from build123d import *

# Parameters (mm, degrees)
SZKIC1_W                    = 22
SZKIC1_H                    = 37
DODANIE_WYCI_GNI_CIE1_DEPTH = 120
SZKIC2_W                    = 42
SZKIC2_H                    = 15
SZKIC2_W_2                  = 15
SZKIC2_H_2                  = 47
WYTNIJ_WYCI_GNI_CIE1_DEPTH  = 112
ZAOKR_GLENIE1_R             = 15
ZAOKR_GLENIE2_R             = 2


with BuildPart() as part:
    # Szkic1 → Dodanie-wyciągnięcie1 (new body)
    with BuildSketch(Plane.XY):
        Polygon((0, 0), (0, 100), (15, 100), (15, 53), (38, 53), (38, 15), (80, 15), (80, 0), align=None)
        with Locations((19, 26.5)):
            Rectangle(SZKIC1_W, SZKIC1_H, mode=Mode.SUBTRACT)
    extrude(amount=DODANIE_WYCI_GNI_CIE1_DEPTH)

    # Szkic2 → Wytnij-wyciągnięcie1 (cut)
    with BuildSketch(Plane.XY.offset(120)):
        with Locations((59, 7.5)):
            Rectangle(SZKIC2_W, SZKIC2_H)
        with Locations((7.5, 76.5)):
            Rectangle(SZKIC2_W_2, SZKIC2_H_2)
    extrude(amount=-WYTNIJ_WYCI_GNI_CIE1_DEPTH, mode=Mode.SUBTRACT)

    # Zaokrąglenie1
    zaokr_glenie1_edges = [part.edges().sort_by_distance(p)[0] for p in [
        (38, 15, 4),
        (15, 53, 4),
    ]]
    fillet(zaokr_glenie1_edges, radius=ZAOKR_GLENIE1_R)

    # Zaokrąglenie2
    zaokr_glenie2_edges = [part.edges().sort_by_distance(p)[0] for p in [
        (38, 26.5, 120),
        (0, 0, 60),
        (38, 53, 60),
        (19, 53, 120),
        (8, 45, 60),
        (8, 26.5, 120),
        (19, 8, 120),
        (30, 26.5, 120),
        (19, 45, 120),
        (19, 0, 120),
        (38, 22.5, 8),
        (38, 0, 64),
        (59, 0, 8),
        (0, 26.5, 120),
        (0, 76.5, 8),
        (0, 53, 64),
        (22.5, 53, 8),
    ]]
    fillet(zaokr_glenie2_edges, radius=ZAOKR_GLENIE2_R)


solid = part.part
Geometry: final body of the model. Coordinates: model frame, mm. A direction names the side the tool comes from. Give positions to 0.01 mm unless a question says otherwise; leave off trailing zeros. Loops run counter-clockwise (first coordinate to the right, second up) from the corner with the lowest first, then second, coordinate; pieces in that order, holes last. Notation, with made-up numbers: M -33.75,59 L -6.75,59 A9 ccw -6.75,69 Z; hole C -33,-14 d2. An arc over 180 degrees is marked long. Put each result on its own line as item: value. Start each with the question number.
1) Contact query for flat-ended pins moving along their axis: pin 1 (24.5 mm diameter, centred on y = 16.5, z = 70.5, fed in from +X); pin 2 (2.5 mm diameter, centred on x = 61.5, z = 5.5, fed in from +Y); pin 3 (8 mm diameter, centred on x = 11.5, z = 98.5, fed in from +Y). Output: stop coordinate, or through.
2) Ray query, line 1 along Y through (x, z) = (18, 109); line 2 along X through (y, z) = (15.5, 66.5); line 3 along X through (y, z) = (81.5, 5). Return the intervals inside material, ascending.
3) Access query for faces 5 (the flat face through (19, 8, 58)), 6 (the flat face through (10, 78, 8)), 7 (the flat face through (66, 15, 4)). Directions: +Z, -Z, +X, -X, +Y, -Y. A direction counts if a zero-diameter tool reaches every point of the face in a straight line with its end or side. Return the directions, or none.
4) Cut plane B-B (x = 13). Output: boundary loops of the cut face in (y, z), then the cut area to 3 significant figures.
5) Pull-direction query (Y, two-part tool) for faces 1 (the cylindrical face through (19.51, 57.28, 3.96)), 2 (the flat face through (8, 25, 58)), 3 (the flat face through (20, 45, 58)), 4 (the flat face through (38, 27, 58)); classes: pulls with the +Y half, pulls with the -Y half, needs draft (parallel to the pull), parting line crosses it, or undercut.
6) Cut plane C-C (z = 39). Output: boundary loops of the cut face in (x, y).
7) Cut plane D-D (y = 59). Output: boundary loops of the cut face in (x, z).
8) Cut plane A-A (y = 32). Output: boundary loops of the cut face in (x, z), then the cut area to 3 significant figures.
Verdict:
1. pin 1: x = 38
1. pin 2: y = 15
1. pin 3: y = 53
2. line 1: 0 to 8, 45 to 53
2. line 2: 0 to 8, 30 to 38
2. line 3: 0 to 15
3. face 5: +Z, -Z
3. face 6: +Z, +X, -X, +Y
3. face 7: +Z, -Z, +X, +Y
4. outline: M 0,0 L 8,0 L 8,118 A2 ccw 6,120 L 2,120 A2 ccw 0,118 Z; M 45,0 L 100,0 L 100,8 L 55,8 A2 cw 53,10 L 53,118 A2 ccw 51,120 L 47,120 A2 ccw 45,118 Z
4. area: 2,290 mm2
5. face 1: pulls with the +Y half
5. face 2: undercut
5. face 3: undercut
5. face 4: needs draft
6. outline: M 0,2 A2 ccw 2,0 L 36,0 A2 ccw 38,2 L 38,51 A2 ccw 36,53 L 2,53 A2 ccw 0,51 Z; hole M 8,8 L 30,8 L 30,45 L 10,45 A2 ccw 8,43 Z
7. outline: M 0,0 L 18,0 L 18,8 L 2,8 A2 ccw 0,6 Z
8. outline: M 0,0 L 8,0 L 8,118 A2 ccw 6,120 L 2,120 A2 ccw 0,118 Z; M 30,0 L 38,0 L 38,118 A2 ccw 36,120 L 32,120 A2 ccw 30,118 Z
8. area: 1,920 mm2
